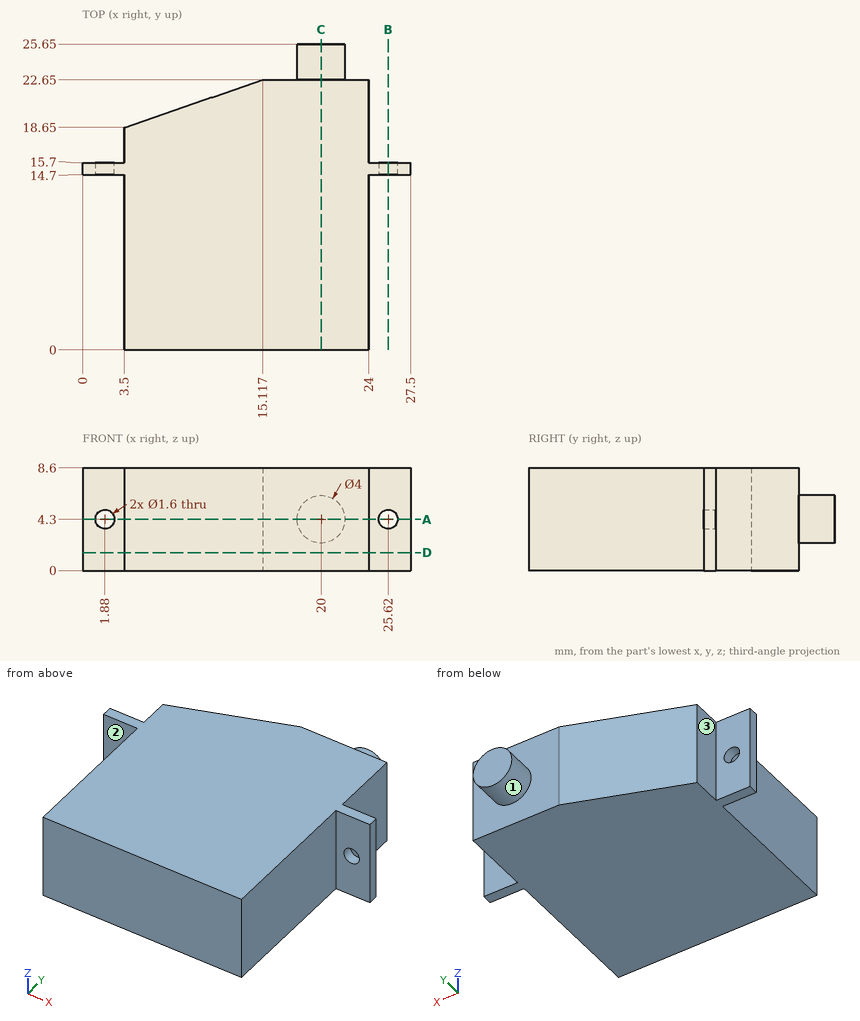
Here's the drawing with two shaded views (mm, measured from the low corner). I have some questions. A direction names the side the tool comes from. Coordinates: 2 decimals unless noted, no trailing zeros. Order: outer loops, then holes, each group sorted by start corner. A loop starts at its lowest first (then second) coordinate and runs counter-clockwise, first axis right, second up. Notation, with made-up numbers: M 55.5,77.5 L 67.5,77.5 A5 cw 67.5,85.5 Z; hole C 88.5,82.25 d9. An arc over 180 degrees is marked long. Answer as CSV lines item,"result".
Item 1: Imagine slicing it at A-A on z = 4.3. Write out the boundary of the cut face in (x, y), plus the area to 3 significant figures.
Results found:
outline,"M 0,14.7 L 1.08,14.7 L 1.08,15.7 L 0,15.7 Z; M 2.68,14.7 L 3.5,14.7 L 3.5,0 L 24,0 L 24,14.7 L 24.82,14.7 L 24.82,15.7 L 24,15.7 L 24,22.65 L 22,22.65 L 22,25.65 L 18,25.65 L 18,22.65 L 15.12,22.65 L 3.5,18.65 L 3.5,15.7 L 2.68,15.7 Z; M 26.42,14.7 L 27.5,14.7 L 27.5,15.7 L 26.42,15.7 Z"
area,"457 mm2"
Item 2: If I drill on line 1 (Z direction, x = 25.62, y = 15.3); line 2 (X direction, y = 18, z = 4.25); line 3 (Y direction, x = 18, z = 6), over which ranges is the centre line in solid material (lowest first)?
Results found:
line 1,"0 to 3.5, 5.1 to 8.6"
line 2,"3.5 to 24"
line 3,"0 to 22.65"
Item 3: Imagine slicing it at D-D on z = 1.5. Write out the boundary of the cut face in (x, y), plus the area to 3 significant figures.
Results found:
outline,"M 0,14.7 L 3.5,14.7 L 3.5,0 L 24,0 L 24,14.7 L 27.5,14.7 L 27.5,15.7 L 24,15.7 L 24,22.65 L 15.12,22.65 L 3.5,18.65 L 3.5,15.7 L 0,15.7 Z"
area,"448 mm2"
Item 4: Imagine slicing it at B-B on x = 25.62. Write out the boundary of the cut face in (y, z).
Results found:
outline,"M 14.7,0 L 15.7,0 L 15.7,3.5 L 14.7,3.5 Z; M 14.7,5.1 L 15.7,5.1 L 15.7,8.6 L 14.7,8.6 Z"
Item 5: On a 3-axis mill with a long thin cutter (end or side, diameter ignored), from which of +Z, -Z, +X, -X, +Y, -Y can I reach the whole of each face in a straight line? I mean the marked faces 1, 2 and 3. Say none if no direction works.
Results found:
face 1,"+Y"
face 2,"+Z, -Z, -X, -Y"
face 3,"+Z, -Z, -X, +Y"
Item 6: Imagine slicing it at C-C on x = 20. Write out the boundary of the cut face in (y, z).
Results found:
outline,"M 0,0 L 22.65,0 L 22.65,2.3 L 25.65,2.3 L 25.65,6.3 L 22.65,6.3 L 22.65,8.6 L 0,8.6 Z"
Item 7: For pin 1 (1.4 mm diameter, centred on x = 25.62, z = 4.3, fed in from -Y); pin 2 (2.5 mm diameter, centred on x = 1.88, z = 4.3, fed in from -Y); pin 3 (0.9 mm diameter, centred on y = 17.5, z = 4.5, fed in from -X); pin 4 (2.5 mm diameter, centred on y = 10, z = 6, fed in from +X), each with a flat end and sliding along its axis, tell me the tip position at first contact or that it passes through.
Results found:
pin 1,"through"
pin 2,"y = 14.7"
pin 3,"x = 3.5"
pin 4,"x = 24"
